from build123d import *

# Parameters (mm, degrees)
F1_DEPTH = 6.985
F2_R     = 5.08


with BuildPart() as f1:
    # F0 (on Front) → F1 (new body)
    with BuildSketch(Plane.XZ):
        with BuildLine():
            Line((16.1311665212, 24.9682), (10.846794214, 15.8153986779))
            Line((10.846794214, 15.8153986779), (19.1199341331, 1.4859))
            Line((19.1199341331, 1.4859), (29.6886787473, 1.4859))
            ThreePointArc((29.6886787473, 1.4859), (16.1311665212, 9.3133333333), (16.1311665212, 24.9682))
        make_face()
        Polygon((9.988909449, 17.3012986779), (10.846794214, 15.8153986779), (16.1311665212, 24.9682), (8.0655832606, 38.9382), (-8.0655832606, 38.9382), (-16.1311665212, 24.9682), (-10.846794214, 15.8153986779), (-9.988909449, 17.3012986779), (-5.5455063073, 17.3012986779), (-9.9719938494, 24.9682), (-4.9859969247, 33.6042), (4.9859969247, 33.6042), (9.9719938494, 24.9682), (5.5455063073, 17.3012986779), align=None)
        with BuildLine():
            Line((-19.1199341331, 1.4859), (-10.846794214, 15.8153986779))
            Line((-10.846794214, 15.8153986779), (-16.1311665212, 24.9682))
            ThreePointArc((-16.1311665212, 24.9682), (-16.1311665212, 9.3133333333), (-29.6886787473, 1.4859))
            Line((-29.6886787473, 1.4859), (-19.1199341331, 1.4859))
        make_face()
        with BuildLine():
            Line((13.5575122262, -26.4541), (8.2731399191, -17.3012986779))
            Line((8.2731399191, -17.3012986779), (-8.2731399191, -17.3012986779))
            Line((-8.2731399191, -17.3012986779), (-13.5575122262, -26.4541))
            ThreePointArc((-13.5575122262, -26.4541), (0, -18.6266666667), (13.5575122262, -26.4541))
        make_face()
        Polygon((9.988909449, -17.3012986779), (8.2731399191, -17.3012986779), (13.5575122262, -26.4541), (29.6886787473, -26.4541), (37.7542620079, -12.4841), (29.6886787473, 1.4859), (19.1199341331, 1.4859), (19.9778188981, 0), (17.7561173272, -3.8481), (26.6090924115, -3.8481), (31.5950893362, -12.4841), (26.6090924115, -21.1201), (16.637098562, -21.1201), (12.2106110199, -13.4531986779), align=None)
        Polygon((-19.9778188981, 0), (-19.1199341331, 1.4859), (-29.6886787473, 1.4859), (-37.7542620079, -12.4841), (-29.6886787473, -26.4541), (-13.5575122262, -26.4541), (-8.2731399191, -17.3012986779), (-9.988909449, -17.3012986779), (-12.2106110199, -13.4531986779), (-16.637098562, -21.1201), (-26.6090924115, -21.1201), (-31.5950893362, -12.4841), (-26.6090924115, -3.8481), (-17.7561173272, -3.8481), align=None)
        with BuildLine():
            ThreePointArc((0, 10.9982), (7.7769018008, 7.7769018008), (10.9982, 0))
            ThreePointArc((10.9982, 0), (10.6234453514, -2.8465438878), (9.5247203206, -5.4991004769))
            Line((9.5247203206, -5.4991004769), (13.5575122262, 1.4859))
            Line((13.5575122262, 1.4859), (19.1199341331, 1.4859))
            Line((19.1199341331, 1.4859), (10.846794214, 15.8153986779))
            Line((10.846794214, 15.8153986779), (8.0655832606, 10.9982))
            Line((8.0655832606, 10.9982), (0, 10.9982))
        make_face()
        Polygon((-5.4919289656, -12.4841), (-9.5247203821, -5.4991003703), (-13.5575122262, 1.4859), (-19.1199341331, 1.4859), (-19.9778188981, 0), (-17.7561173272, -3.8481), (-16.637098562, -3.8481), (-11.6511016373, -12.4841), (-12.2106110199, -13.4531986779), (-9.988909449, -17.3012986779), (-8.2731399191, -17.3012986779), align=None)
        with BuildLine():
            ThreePointArc((-9.5247203821, -5.4991003703), (-9.5247207028, 5.4990998148), (0, 10.9982))
            Line((0, 10.9982), (-8.0655832606, 10.9982))
            Line((-8.0655832606, 10.9982), (-10.846794214, 15.8153986779))
            Line((-10.846794214, 15.8153986779), (-19.1199341331, 1.4859))
            Line((-19.1199341331, 1.4859), (-13.5575122262, 1.4859))
            Line((-13.5575122262, 1.4859), (-9.5247203821, -5.4991003703))
        make_face()
        Polygon((13.5575122262, 1.4859), (9.5247203206, -5.4991004769), (5.4919289656, -12.4841), (8.2731399191, -17.3012986779), (9.988909449, -17.3012986779), (12.2106110199, -13.4531986779), (11.6511016373, -12.4841), (16.637098562, -3.8481), (17.7561173272, -3.8481), (19.9778188981, 0), (19.1199341331, 1.4859), align=None)
        Polygon((-8.0655832606, 10.9982), (0, 10.9982), (8.0655832606, 10.9982), (10.846794214, 15.8153986779), (9.988909449, 17.3012986779), (5.5455063073, 17.3012986779), (4.9859969247, 16.3322), (-4.9859969247, 16.3322), (-5.5455063073, 17.3012986779), (-9.988909449, 17.3012986779), (-10.846794214, 15.8153986779), align=None)
        with BuildLine():
            Line((5.4919289656, -12.4841), (9.5247203206, -5.4991004769))
            ThreePointArc((9.5247203206, -5.4991004769), (-6.15e-08, -10.9982), (-9.5247203821, -5.4991003703))
            Line((-9.5247203821, -5.4991003703), (-5.4919289656, -12.4841))
            Line((-5.4919289656, -12.4841), (-8.2731399191, -17.3012986779))
            Line((-8.2731399191, -17.3012986779), (8.2731399191, -17.3012986779))
            Line((8.2731399191, -17.3012986779), (5.4919289656, -12.4841))
        make_face()
    extrude(amount=F1_DEPTH)

    # F2
    f2_edges = [f1.edges().sort_by_distance(p)[0] for p in [
        (16.131167, -3.4925, 24.9682),
        (-8.065583, -3.4925, 38.9382),
        (8.065583, -3.4925, 38.9382),
        (-16.131167, -3.4925, 24.9682),
        (-29.688679, -3.4925, 1.4859),
        (-37.754262, -3.4925, -12.4841),
        (-13.557512, -3.4925, -26.4541),
        (-29.688679, -3.4925, -26.4541),
        (13.557512, -3.4925, -26.4541),
        (29.688679, -3.4925, -26.4541),
        (37.754262, -3.4925, -12.4841),
        (29.688679, -3.4925, 1.4859),
    ]]
    fillet(f2_edges, radius=F2_R)


solid = f1.part
Design review of the part built by this model. Coordinates are the model's own, in mm. A direction names the side the tool comes from. Coordinates: 2 decimals unless noted, no trailing zeros. Loops run counter-clockwise (first coordinate to the right, second up) from the corner with the lowest first, then second, coordinate; pieces in that order, holes last.
Item 1: Wall thickness on L1, parallel to X at y = -4.25, z = -10; L2, parallel to X at y = -1.5, z = -16.5; L3, parallel to X at y = -1.75, z = -13: over which ranges is each line inside the solid? List them lowest first.
Completed:
L1: x = -36.32 to -30.16, -13.09 to -4.58, 4.58 to 13.09, 30.16 to 36.32
L2: x = -35.44 to -29.28, -13.97 to 13.97, 29.28 to 35.44
L3: x = -36.94 to -31.3, -11.95 to 11.95, 31.3 to 36.94
Item 2: Add section A-A (z = 6). Write out the cut boundary in (x, y) (3 decimals), and give its area (3 significant figures).
Completed:
outline: (-18.691, -6.985) - (-9.217, -6.985) - (-9.217, 0) - (-18.691, 0) - close; (9.217, -6.985) - (18.691, -6.985) - (18.691, 0) - (9.217, 0) - close
area: 132 mm2
Item 3: Add section B-B (x = -28.5). Write out the cut boundary in (y, z) (3 decimals), and give its area (3 significant figures).
Completed:
outline: (-6.985, -26.145) - (0, -26.145) - (0, -17.845) - (-6.985, -17.845) - close; (-6.985, -7.123) - (0, -7.123) - (0, 1.355) - (-6.985, 1.355) - close
area: 117 mm2
Item 4: For faces 4 (the cylindrical face through (13.992, -3.541, -25.936)), 5 (the flat face through (-12.13, -3.44, 31.9)), 6 (the flat face through (22, -3, -3.848)), list the 3-axis set-ups (+Z, -Z, +X, -X, +Y, -Y) from which the entire face can be reached by the end or side of a thin tool; tool diameter is ignored.
Completed:
face 4: -Z, +Y, -Y
face 5: +Z, -X, +Y, -Y
face 6: +Y, -Y
Item 5: Draft analysis for pull direction Z (two halves, no side actions). For faces 1 (the cylindrical face through (15.465, -3.541, 25.085)), 2 (the cylindrical face through (-36.97, -3.54, -12.45)), 3 (the flat face through (12.2, -3.44, 31.78)), state which applies: pulls with the +Z half, pulls with the -Z half, needs draft (parallel to the pull), parting line crosses it, or undercut.
Completed:
face 1: undercut
face 2: parting line crosses it
face 3: pulls with the +Z half
Item 6: Add section D-D (x = 2.5). Write out the cut boundary in (y, z) (3 decimals), and give its area (3 significant figures).
Completed:
outline: (-6.985, -18.828) - (0, -18.828) - (0, -10.71) - (-6.985, -10.71) - close; (-6.985, 10.71) - (0, 10.71) - (0, 16.332) - (-6.985, 16.332) - close; (-6.985, 33.604) - (0, 33.604) - (0, 38.938) - (-6.985, 38.938) - close
area: 133 mm2
Item 7: Clearance check with a flat-ended pin moving along its axis: pin 1 (2 mm diameter, centred on x = 2.5, y = -4.5, fed in from -Z). State where the tip first meets the part, or that it passes through.
Completed:
pin 1: stops at z = -19.02
Item 8: Add section C-C (z = -16). Write out the cut boundary in (x, y) (3 decimals).
Completed:
outline: (-35.724, -6.985) - (-29.565, -6.985) - (-29.565, 0) - (-35.724, 0) - close; (-13.681, -6.985) - (13.681, -6.985) - (13.681, 0) - (-13.681, 0) - close; (29.565, -6.985) - (35.724, -6.985) - (35.724, 0) - (29.565, 0) - close
